CAD build for the part. Positions are in the model's coordinates, mm. A direction names the side the tool comes from. Give positions to 0.01 mm unless a question says otherwise; leave off trailing zeros. Use one line per item in the form item = value.
```python
from build123d import *

# Parameters (mm, degrees)
SKETCH_2_W             = 350
SKETCH_2_H             = 310
EXTRUDE_1_DEPTH        = 15
SKETCH_3_R             = 3
CUT_EXTRUDE_1_DEPTH    = 468.787344848
SKETCH_4_R             = 5.5
CUT_EXTRUDE_2_DEPTH    = 6
HOLE_WIZARD_M8_1_D     = 6.8
HOLE_WIZARD_M8_1_DEPTH = 19.75
HOLE_WIZARD_M8_1_TIP   = 2.042926105


with BuildPart() as part:
    # 草图2 → 凸台-拉伸1 (new body)
    with BuildSketch(Plane(origin=(0, 0, 0), x_dir=(1, 0, 0), z_dir=(0, 1, 0))):
        with Locations((175, 155)):
            Rectangle(SKETCH_2_W, SKETCH_2_H)
    extrude(amount=EXTRUDE_1_DEPTH)

    # 草图3 → 切除-拉伸1 (cut, through all)
    with BuildSketch(Plane(origin=(0, 15, 0), x_dir=(1, 0, 0), z_dir=(0, 1, 0))):
        with Locations(Location((342, 292, 0), (0, 0, 270))):
            Circle(SKETCH_3_R)
        with Locations(Location((342, 268, 0), (0, 0, 270))):
            Circle(SKETCH_3_R)
        with Locations(Location((342, 42, 0), (0, 0, 90))):
            Circle(SKETCH_3_R)
        with Locations(Location((342, 18, 0), (0, 0, 90))):
            Circle(SKETCH_3_R)
        with Locations(Location((8, 18, 0), (0, 0, 270))):
            Circle(SKETCH_3_R)
        with Locations(Location((8, 42, 0), (0, 0, 270))):
            Circle(SKETCH_3_R)
        with Locations(Location((8, 268, 0), (0, 0, 90))):
            Circle(SKETCH_3_R)
        with Locations(Location((8, 292, 0), (0, 0, 90))):
            Circle(SKETCH_3_R)
    extrude(amount=-CUT_EXTRUDE_1_DEPTH, mode=Mode.SUBTRACT)

    # 草图4 → 切除-拉伸2 (cut)
    with BuildSketch(Plane(origin=(0, 15, 0), x_dir=(1, 0, 0), z_dir=(0, 1, 0))):
        with Locations(Location((342, 292, 0), (0, 0, 270))):
            Circle(SKETCH_4_R)
        with Locations(Location((342, 268, 0), (0, 0, 270))):
            Circle(SKETCH_4_R)
        with Locations(Location((342, 42, 0), (0, 0, 90))):
            Circle(SKETCH_4_R)
        with Locations(Location((342, 18, 0), (0, 0, 90))):
            Circle(SKETCH_4_R)
        with Locations(Location((8, 18, 0), (0, 0, 270))):
            Circle(SKETCH_4_R)
        with Locations(Location((8, 42, 0), (0, 0, 270))):
            Circle(SKETCH_4_R)
        with Locations(Location((8, 268, 0), (0, 0, 90))):
            Circle(SKETCH_4_R)
        with Locations(Location((8, 292, 0), (0, 0, 90))):
            Circle(SKETCH_4_R)
    extrude(amount=-CUT_EXTRUDE_2_DEPTH, mode=Mode.SUBTRACT)

    # M8 螺纹孔1
    with Locations(Plane(origin=(50, 15, -230), x_dir=(0, 0, 1), z_dir=(0, 1, 0))):
        with Locations((0, 0), (0, 50), (40, 0), (40, 50), (40, 90), (40, 160), (0, 200), (0, 250), (40, 250), (40, 200), (110, 0), (110, 50), (110, 90), (110, 160), (110, 200), (110, 250), (150, 250), (150, 200), (150, 50), (150, 0)):
            Hole(HOLE_WIZARD_M8_1_D / 2, depth=HOLE_WIZARD_M8_1_DEPTH)
            with Locations((0, 0, -(HOLE_WIZARD_M8_1_DEPTH + HOLE_WIZARD_M8_1_TIP / 2))):  # 118° drill point
                Cone(0, HOLE_WIZARD_M8_1_D / 2, HOLE_WIZARD_M8_1_TIP, mode=Mode.SUBTRACT)


solid = part.part
```
1. Drop flat-ended pins along their axis: P1, Ø3.5, axis at x = 343, z = -268, coming from the +Y side; P2, Ø5.5, axis at x = 6.5, z = -18.5, coming from the +Y side. Give the stop position or say it passes through.
Result sheet:
P1 = through
P2 = 9
2. Tool access for faces 1 (the flat face through (339.6, 9, -289.6)), 2 (the flat face through (173, 7, -310)): list every direction of +Z, -Z, +X, -X, +Y, -Y with a clear straight run to the whole face (end or side of a thin tool).
Result sheet:
face_1 = +Y
face_2 = -Z, +X, -X, +Y, -Y
3. Drill centre lines: line 1 (Z direction, x = 300, y = 9.75); line 2 (Z direction, x = 342, y = 11.1); line 3 (X direction, y = 10.5, z = -230). Where is each one in solid material? Low to high.
Result sheet:
line_1 = -310 to -233.4, -226.6 to -193.4, -186.6 to -123.4, -116.6 to -83.4, -76.6 to 0
line_2 = -310 to -297.5, -286.5 to -273.5, -262.5 to -47.5, -36.5 to -23.5, -12.5 to 0
line_3 = 0 to 46.6, 53.4 to 96.6, 103.4 to 246.6, 253.4 to 296.6, 303.4 to 350
4. Mould opens along Z. For faces 3 (the cylindrical face through (339.89, 12.04, -286.92)), 4 (the flat face through (0, 7, -153)), 5 (the flat face through (173, 7, 0)) say: pulls with the +Z half, pulls with the -Z half, needs draft (parallel to the pull), parting line crosses it, or undercut.
Result sheet:
face_3 = undercut
face_4 = needs draft
face_5 = pulls with the +Z half
